from build123d import *

# Parameters (mm, degrees)
BASE_FLANGE1_DEPTH = 644.525
SKETCH3_R          = 3.429
CUT_EXTRUDE1_DEPTH = 3.175
SKETCH5_R          = 3.429
SKETCH5_R_2        = 9.525
CUT_EXTRUDE2_DEPTH = 3.175
FILLET1_R          = 3.175


# Read off the part's stored shape, not the designer's step: Base-Flange1
with BuildPart() as part:
    # Base-Flange1 outline → Base-Flange1 (new body)
    with BuildSketch(Plane(origin=(0, 0, 0), x_dir=(0, 0, -1), z_dir=(1, 0, 0))):
        with BuildLine():
            Line((3.175, 6.35), (3.175, 44.45))
            Line((3.175, 44.45), (0, 44.45))
            Line((0, 44.45), (0, 6.35))
            ThreePointArc((0, 6.35), (1.859871939, 1.859871939), (6.35, 0))
            Line((6.35, 0), (53.975, 0))
            Line((53.975, 0), (53.975, 3.175))
            Line((53.975, 3.175), (6.35, 3.175))
            ThreePointArc((6.35, 3.175), (4.10493597, 4.10493597), (3.175, 6.35))
        make_face()
    extrude(amount=BASE_FLANGE1_DEPTH)

    # Sketch3 → Cut-Extrude1 (cut)
    with BuildSketch(Plane.XZ):
        with Locations(Location((631.825, -19.05, 0), (0, 0, 270))):
            Circle(SKETCH3_R)
        with Locations(Location((631.825, -38.1, 0), (0, 0, 270))):
            Circle(SKETCH3_R)
        with Locations(Location((12.7, -38.1, 0), (0, 0, 270))):
            Circle(SKETCH3_R)
        with Locations(Location((12.7, -19.05, 0), (0, 0, 270))):
            Circle(SKETCH3_R)
    extrude(amount=-CUT_EXTRUDE1_DEPTH, mode=Mode.SUBTRACT)

    # Sketch5 → Cut-Extrude2 (cut)
    with BuildSketch(Plane.XY):
        with Locations((631.825, 28.575)):
            Circle(SKETCH5_R)
        with Locations((6.35, 31.75)):
            Circle(SKETCH5_R)
        with Locations((63.5, 28.575)):
            Circle(SKETCH5_R_2)
        with Locations((25.4, 31.75)):
            Circle(SKETCH5_R)
    extrude(amount=-CUT_EXTRUDE2_DEPTH, mode=Mode.SUBTRACT)

    # Fillet1
    fillet1_edges = [part.edges().sort_by_distance(p)[0] for p in [
        (644.525, 1.5875, -53.975),
        (0, 1.5875, -53.975),
        (644.525, 44.45, -1.5875),
        (0, 44.45, -1.5875),
    ]]
    fillet(fillet1_edges, radius=FILLET1_R)


solid = part.part
Could you check a few things on this model? Use its own coordinates, in mm. A direction names the side the tool comes from. Coordinates: 2 decimals unless noted, no trailing zeros. Order: outer loops, then holes, each group sorted by start corner. A loop starts at its lowest first (then second) coordinate and runs counter-clockwise, first axis right, second up. Notation, with made-up numbers: (4, -38) -> (62, -38) arc R34 cw to (62, -7) -> close; hole circle Ø5 at (-5, 84.5). An arc over 180 degrees is marked (long way). One line per item, written item: value. Start each with the question number.
1) Imagine slicing it at B-B on y = 13. List the corners of the cut face in (x, z) for me (3 decimals), plus the area to 3 significant figures.
2) If I drill on L1, parallel to Z at x = 12, y = 1 (3 decimals); L2, parallel to Y at x = 150.5, z = -36 (3 decimals); L3, parallel to Z at x = 584.5, y = 39.5 (3 decimals), over which ranges is the centre line in solid material (lowest first)? Write a range as [from, to].
3) We'd pull the mould along X, two halves only. Please class faces 1 (the flat face through (0, 2, -14)), 2 (the flat face through (318, 0, -30)), 3 (the cylindrical face through (72.585, 31.436, -1.565)), 4 (the flat face through (644.525, 2, -14)): +X half, -X half, draft (parallel to the pull), parting line (faces both ways), or undercut.
4) Imagine slicing it at A-A on x = 63.5. List the corners of the cut face in (y, z) for me (3 decimals), plus the area to 3 significant figures.
5) Which directions (+Z, -Z, +X, -X, +Y, -Y) give clear straight access to the entire face, cutting with the end or side of a thin tool? Please do faces 5 (the flat face through (318, 26, 0)), 6 (the flat face through (318, 25, -3.175)).
6) I'm going to push flat-ended pins straight in: pin 1 (4 mm diameter, centred on x = 555.5, z = -30, fed in from +Y) (3 decimals); pin 2 (8 mm diameter, centred on x = 281.5, y = 31.5, fed in from -Z) (3 decimals); pin 3 (5.5 mm diameter, centred on x = 12.7, z = -38.1, fed in from +Y). Where does each tip first touch, or does it pass through?
Answer list:
1. outline: (0, -3.175) -> (644.525, -3.175) -> (644.525, 0) -> (0, 0) -> close
1. area: 2,050 mm2
2. L1: z = [-53.975, -41.457], [-34.743, -22.407], [-15.693, -2.929]
2. L2: y = [0, 3.175]
2. L3: z = [-3.175, 0]
3. face 1: -X half
3. face 2: draft
3. face 3: undercut
3. face 4: +X half
4. outline: (0, -53.975) -> (3.175, -53.975) -> (3.175, -6.35) arc R3.175 cw to (6.35, -3.175) -> (19.05, -3.175) -> (19.05, 0) -> (6.35, 0) arc R6.35 ccw to (0, -6.35) -> close; (38.1, -3.175) -> (44.45, -3.175) -> (44.45, 0) -> (38.1, 0) -> close
4. area: 235 mm2
5. face 5: +Z, +X, -X, +Y, -Y
5. face 6: -Z, +X, -X, +Y
6. pin 1: stops at y = 3.175
6. pin 2: stops at z = -3.175
6. pin 3: passes through
